Work out the finished part from the listing and answer in its coordinate system (mm). Face numbers are marked on the shaded views. A direction names the side the tool comes from. Round coordinates to 2 decimals unless told otherwise and drop trailing zeros. Order: outer loops, then holes, each group sorted by start corner. A loop starts at its lowest first (then second) coordinate and runs counter-clockwise, first axis right, second up.
from build123d import *

# Parameters (mm, degrees)
F7_DEPTH  = 10
F8_R      = 1
F10_D     = 3.2
F12_D     = 3.2
F13_DEPTH = 2
F15_DEPTH = 3
F17_DEPTH = 2


with BuildPart() as f7:
    # F6 (on Front) → F7 (new body, symmetric)
    with BuildSketch(Plane.XZ):
        with BuildLine():
            Line((0, 3), (0, 0))
            Line((0, 0), (21.025, 0))
            Line((21.025, 0), (21.025, 4))
            Line((21.025, 4), (11.625, 4))
            Line((11.625, 4), (11.625, 10.625))
            ThreePointArc((11.625, 10.625), (9.9769265057, 16.5917044924), (5.5, 20.8666124219))
            Line((5.5, 20.8666124219), (5.5, 30.2666124219))
            Line((5.5, 30.2666124219), (0.75, 30.2666124219))
            Line((0.75, 30.2666124219), (0.75, 18.2130251054))
            ThreePointArc((0.75, 18.2130251054), (7.6157506665, 10.2495445623), (0, 3))
        make_face()
    extrude(amount=F7_DEPTH, both=True)

    # F8
    f8_edges = [f7.edges().sort_by_distance(p)[0] for p in [
        (0.75, 0, 18.213025),
        (5.5, 0, 30.266612),
        (5.5, 0, 20.866612),
        (11.625, 0, 4),
        (11.625, 0, 10.625),
        (21.025, 0, 4),
        (0.75, 0, 30.266612),
    ]]
    fillet(f8_edges, radius=F8_R)

    # F10 (through all)
    with Locations(Plane.YZ.offset(5.5)):
        with Locations((-5, 25.3573823446), (5, 25.3573823446)):
            Hole(F10_D / 2)

    # F12 (through all)
    with Locations(Plane.XY.offset(4)):
        with Locations((16.325, 5), (16.325, -5)):
            Hole(F12_D / 2)

    # F11 (on face) → F13 (cut)
    with BuildSketch(Plane.XY.offset(4)):
        Polygon((16.325, 8.1), (13.6403212483, 6.55), (13.6403212483, 3.45), (16.325, 1.9), (19.0096787517, 3.45), (19.0096787517, 6.55), align=None)
        Polygon((16.325, -1.9), (13.6403212483, -3.45), (13.6403212483, -6.55), (16.325, -8.1), (19.0096787517, -6.55), (19.0096787517, -3.45), align=None)
    extrude(amount=-F13_DEPTH, mode=Mode.SUBTRACT)

    # F14 (on face) → F15 (join)
    with BuildSketch(Plane(origin=(0, 0, 0), x_dir=(1, 0, 0), z_dir=(0, 0, -1))):
        with BuildLine():
            Line((0, 14), (0, 10))
            Line((0, 10), (2, 10))
            Line((2, 10), (2, 12))
            ThreePointArc((2, 12), (3, 13), (2, 14))
            Line((2, 14), (0, 14))
        make_face()
        with BuildLine():
            Line((21.025, 2), (21.025, 0))
            Line((21.025, 0), (25.025, 0))
            Line((25.025, 0), (25.025, 2))
            ThreePointArc((25.025, 2), (24.025, 3), (23.025, 2))
            Line((23.025, 2), (21.025, 2))
        make_face()
        with BuildLine():
            Line((25.025, 0), (21.025, 0))
            Line((21.025, 0), (21.025, -2))
            Line((21.025, -2), (23.025, -2))
            ThreePointArc((23.025, -2), (24.025, -3), (25.025, -2))
            Line((25.025, -2), (25.025, 0))
        make_face()
    extrude(amount=-F15_DEPTH)

    # F16: F7 across plane


with BuildPart() as f7_1:
    add(f7.part)
    add(f7.part.mirror(Plane.YZ))

    # F9 (on face) → F17 (cut)
    with BuildSketch(Plane.YZ.offset(5.5)):
        Polygon((-1.9, 25.3573823446), (-3.45, 28.0420610963), (-6.55, 28.0420610963), (-8.1, 25.3573823446), (-6.55, 22.6727035928), (-3.45, 22.6727035928), align=None)
        Polygon((6.55, 28.0420610963), (3.45, 28.0420610963), (1.9, 25.3573823446), (3.45, 22.6727035928), (6.55, 22.6727035928), (8.1, 25.3573823446), align=None)
    extrude(amount=-F17_DEPTH, mode=Mode.SUBTRACT)


solid = f7_1.part
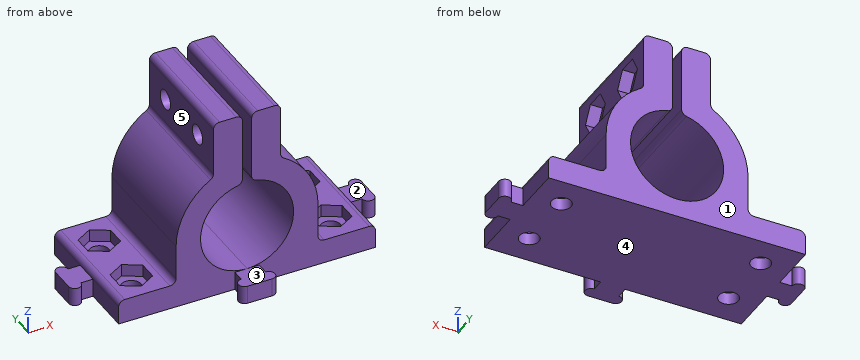
Item 1: A tool of negligible diameter and unlimited length cuts with its end or side. For the marked faces 1, 2, 3, 4 and 5, from which of +Z, -Z, +X, -X, +Y, -Y can it reach the whole face along a straight path? Write none if from no direction.
Item 2: Find section A-A (z = 10). Write down the section's boundary in (x, y) (3 decimals).
Item 3: Given pin 1 (0.6 mm diameter, centred on y = -5.5, z = 3.5, fed in from -X); pin 2 (1 mm diameter, centred on y = -6, z = 13, fed in from +X); pin 3 (2 mm diameter, centred on x = 17.5, y = -8, fed in from +Z); pin 4 (3 mm diameter, centred on x = -9, y = 7.5, fed in from -Z), each flat-ended and moving along its own axis, determine where each tip first touches the part or whether it passes through.
Item 4: Find section C-C (y = -5). State how many separate pieces and enclosed holes the cut face has, plus the area to 3 significant figures.
Item 5: Find the intervals of material crossed by line 1 along Y through (x, z) = (-2, 25); line 2 along X through (y, z) = (-7.5, 2.5) (3 decimals); line 3 along Z through (x, y) = (-3.8, 5), in increasing order.
Item 6: Find section D-D (z = 6.5). Write down the section's boundary in (x, y) (3 decimals), plus the area to 3 significant figures.
Model answer:
1. face 1: +Z, -Z, +X, -X, +Y
1. face 2: +Z, +X, +Y, -Y
1. face 3: +Z, +X, -X, -Y
1. face 4: -Z, +X, -X, +Y, -Y
1. face 5: +Z, -X, +Y, -Y
2. outline: (-11.625, -10) - (-7.599, -10) - (-7.599, 10) - (-11.625, 10) - close; (7.599, -10) - (11.625, -10) - (11.625, 10) - (7.599, 10) - close
3. pin 1: stops at x = -21
3. pin 2: stops at x = 11.47
3. pin 3: stops at z = 4
3. pin 4: stops at z = 0
4. separate pieces: 5
4. enclosed holes: 0
4. area: 357 mm2
5. line 1: y = -10 to -6.56, -3.44 to 3.44, 6.56 to 10
5. line 2: x = -21.025 to -17.364, -15.286 to 15.286, 17.364 to 21.025
5. line 3: z = 0 to 4.01, 17.24 to 23.76, 26.96 to 30.27
6. outline: (-11.625, -10) - (-6.413, -10) - (-6.413, 10) - (-11.625, 10) - close; (6.413, -10) - (11.625, -10) - (11.625, 10) - (6.413, 10) - close
6. area: 208 mm2
